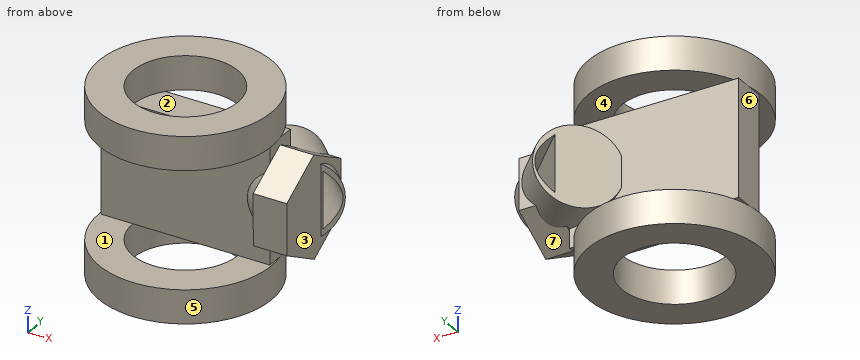
from build123d import *

# Parameters (mm, degrees)
SKETCH_1_W           = 50.17161873
SKETCH_1_H           = 34.913239838
EXTRUDE_1_DEPTH      = 10
SKETCH_2_R           = 25.596904926
SKETCH_2_R_2         = 15.596904926
EXTRUDE_1_2_DEPTH    = 10
EXTRUDE_START        = 10
SKETCH_3_R           = 25.596904926
SKETCH_3_R_2         = 15.596904926
EXTRUDE_2_DEPTH      = 10
EXTRUDE_2_2_DEPTH    = 10
EXTRUDE_3_DEPTH      = 7
EXTRUDE_3_DEPTH_BACK = 12
SKETCH_5_R           = 12.097292752
CUT_EXTRUDE_1_DEPTH  = 63.060098254


with BuildPart() as part:
    # 草圖1 → Extrude 1 (new body)
    with BuildSketch(Plane(origin=(0, 0, 0), x_dir=(1, 0, 0), z_dir=(0, 1, 0))):
        Rectangle(SKETCH_1_W, SKETCH_1_H)
    extrude(amount=EXTRUDE_1_DEPTH)

    # 草圖2 → Extrude 1 2 (add)
    with BuildSketch(Plane.XY.offset(17.456619919)):
        Circle(SKETCH_2_R)
        Circle(SKETCH_2_R_2, mode=Mode.SUBTRACT)
    extrude(amount=EXTRUDE_1_2_DEPTH)

    # 草圖3 → Extrude 2 (add)
    with BuildSketch(Plane(origin=(0, 0, -17.456619919), x_dir=(-1, 0, 0), z_dir=(0, 0, -1)).offset(EXTRUDE_START)):
        Circle(SKETCH_3_R)
        Circle(SKETCH_3_R_2, mode=Mode.SUBTRACT)
    extrude(amount=-EXTRUDE_2_DEPTH)

    # 草圖4 → Extrude 2 2 (add)
    with BuildSketch(Plane(origin=(25.085809365, 0, 0), x_dir=(0, 0, -1), z_dir=(1, 0, 0))):
        Polygon((7.767540636, -8.142290403), (15.342896504, 5.2005267), (7.575355868, 18.432385876), (-7.767540636, 18.321427949), (-15.342896504, 4.978610845), (-7.575355868, -8.253248331), align=None)
    extrude(amount=EXTRUDE_2_2_DEPTH)

    # 草圖5 → 填料-伸長3 (add, two sides: drawn at the far end of the back side and taken through both)
    with BuildSketch(Plane(origin=(8.35434404, -8.354125583, -0.060416002), x_dir=(-0.003615890802849244, 0.003615796250954227, -0.9999869255901167), z_dir=(0.7071067811865482, -0.7070882910578936, -0.005113574955600474)).offset(-EXTRUDE_3_DEPTH_BACK)):
        with Locations((-0.42297231, 25.100981723)):
            Circle(SKETCH_5_R)
    extrude(amount=EXTRUDE_3_DEPTH + EXTRUDE_3_DEPTH_BACK)

    # 草圖6 → 除料-伸長1 (cut, through all)
    with BuildSketch(Plane(origin=(13.304091508, -13.30374362, -0.096211026), x_dir=(-0.0036158908028492477, 0.0036157962509542232, -0.9999869255901167), z_dir=(0.7071067811865483, -0.7070882910578935, -0.005113574955600474))):
        with BuildLine():
            Line((-8.90297564, 31.358512716), (8.125719102, 31.358512716))
            add(Edge.make_bspline(
                [(8.125719102, 31.358512716), (-0.388628269, 41.854112763), (-8.90297564, 31.358512716)],
                knots=[0, 0, 0, 1, 1, 1], degree=2))
        make_face()
    extrude(amount=-CUT_EXTRUDE_1_DEPTH, mode=Mode.SUBTRACT)


solid = part.part
Verification items for the finished model (mm, model axes). Face numbers are marked on the shaded views. A direction names the side the tool comes from. Give positions to 0.01 mm unless a question says otherwise; leave off trailing zeros. Order: outer loops, then holes, each group sorted by start corner. A loop starts at its lowest first (then second) coordinate and runs counter-clockwise, first axis right, second up. Notation, with made-up numbers: M -15,71 L -4,71 A24 ccw -4,82 Z; hole C -11,68 d9. An arc over 180 degrees is marked long. Use one line per item in the form item = value. Start each with the question number.
Q1. Section check C-C (x = 13). Count the separate pieces of the cut face and the enclosed holes in it, then the cut area to 3 significant figures.
Q2. Access from +Z, -Z, +X, -X, +Y, -Y to the whole of each face (thin tool, end or side, straight path). Record for the marked faces 5, 6 and 7.
Q3. Mould release check, pull along Z, two halves, no side actions. Record for the marked faces 1, 2, 3 and 4: +Z half, -Z half, draft (parallel to the pull), parting line (faces both ways), or undercut.
Q4. Section check D-D (x = -8). Enter the section's corners in (y, z), then the cut area to 3 significant figures.
Q5. Scan lines: line 1 along X through (y, z) = (0, 19.5); line 2 along Z through (x, y) = (1.5, 17.5). Record each from-to range of solid material in increasing order. Write a range as [from, to].
Q6. Section check B-B (y = 7). Enter the section's corners in (x, z).
Q7. Go/stop test with flat-tipped pins: pin 1 Ø18.5 at (x, y) = (0, 0) entering from -Z; pin 2 Ø5 at (x, z) = (-7.5, 10) entering from -Y; pin 3 Ø3 at (y, z) = (5.5, -5) entering from -X. Record where each tip stops, or that it passes through.
Q8. Section check A-A (x = 0). Enter the section's corners in (y, z), then the cut area to 3 significant figures.
Evaluation:
q1.separate_pieces = 3
q1.enclosed_holes = 0
q1.area = 947 mm2
q2.face_5 = -Z
q2.face_6 = -X, +Y, -Y
q2.face_7 = -Z, +X, +Y
q3.face_1 = undercut
q3.face_2 = +Z half
q3.face_3 = draft
q3.face_4 = undercut
q4.outline = M -24.31,-27.46 L -13.39,-27.46 L -13.39,-17.46 L -24.31,-17.46 Z; M -24.31,17.46 L -13.39,17.46 L -13.39,27.46 L -24.31,27.46 Z; M 0,-17.46 L 10,-17.46 L 10,17.46 L 0,17.46 Z; M 13.39,-27.46 L 24.31,-27.46 L 24.31,-17.46 L 13.39,-17.46 Z; M 13.39,17.46 L 24.31,17.46 L 24.31,27.46 L 13.39,27.46 Z
q4.area = 786 mm2
q5.line_1 = [-25.6, -15.6], [15.6, 25.6]
q5.line_2 = [-27.46, -17.46], [17.46, 27.46]
q6.outline = M -25.09,-17.46 L -24.62,-17.46 L -24.62,-27.46 L -13.94,-27.46 L -13.94,-17.46 L 13.94,-17.46 L 13.94,-27.46 L 24.62,-27.46 L 24.62,-17.46 L 25.09,-17.46 L 25.09,-14.29 L 35.09,-14.29 L 35.09,14.2 L 25.09,14.2 L 25.09,17.46 L 24.62,17.46 L 24.62,27.46 L 13.94,27.46 L 13.94,17.46 L -13.94,17.46 L -13.94,27.46 L -24.62,27.46 L -24.62,17.46 L -25.09,17.46 Z
q7.pin_1 = -17.46
q7.pin_2 = 0
q7.pin_3 = -25.09
q8.outline = M -25.6,-27.46 L -15.6,-27.46 L -15.6,-17.46 L -25.6,-17.46 Z; M -25.6,17.46 L -15.6,17.46 L -15.6,27.46 L -25.6,27.46 Z; M 0,-17.46 L 10,-17.46 L 10,17.46 L 0,17.46 Z; M 15.6,-27.46 L 25.6,-27.46 L 25.6,-17.46 L 15.6,-17.46 Z; M 15.6,17.46 L 25.6,17.46 L 25.6,27.46 L 15.6,27.46 Z
q8.area = 749 mm2
